from build123d import *

# Parameters (mm, degrees)
F1_DEPTH = 76.2
F2_W     = 17.6722221076
F2_H     = 9.8298916579
F2_W_2   = 18.5227831721
F3_DEPTH = 76.2
F4_R     = 3.4516477469
F4_R_2   = 3.5094678627
F5_DEPTH = 127
F6_R     = 3.428244009
F7_DEPTH = 127


with BuildPart() as f1:
    # F0 (on Right) → F1 (new body)
    with BuildSketch(Plane.YZ):
        with BuildLine():
            Line((-43.5515455902, 4.9651595764), (-39.2007894463, -3.8494697966))
            ThreePointArc((-39.2007894463, -3.8494697966), (59.7212641248, -33.7173735079), (95.7566574216, 63.1284564734))
            Line((95.7566574216, 63.1284564734), (82.136558344, 69.8877791238))
            Line((82.136558344, 69.8877791238), (86.031280458, 60.8586706221))
            ThreePointArc((86.031280458, 60.8586706221), (50.4707031722, -26.2634284737), (-35.969786346, 10.9233511612))
            Line((-35.969786346, 10.9233511612), (-43.5515455902, 4.9651595764))
        make_face()
    extrude(amount=F1_DEPTH)

    # F2 (on face) → F3 (join)
    with BuildSketch(Plane(origin=(0, -33.0492176978, -16.3125505187), x_dir=(1, 0, 0), z_dir=(0, -0.8967168388, -0.4426046894))):
        with Locations((8.8361110538, 18.8135146783)):
            Rectangle(F2_W, F2_H)
        with Locations((66.9386084139, 18.8135146783)):
            Rectangle(F2_W_2, F2_H)
    extrude(amount=F3_DEPTH)

    # F4 (on face) → F5 (cut)
    with BuildSketch(Plane.YZ.offset(76.2)):
        with Locations((-79.3107077479, -18.0164370686)):
            Circle(F4_R)
        with Locations((-95.9507897496, -26.2444168329)):
            Circle(F4_R_2)
    extrude(amount=-F5_DEPTH, mode=Mode.SUBTRACT)

    # F6 (on face) → F7 (cut)
    with BuildSketch(Plane.YZ.offset(76.2)):
        with Locations((-63.4221956134, -10.355903767)):
            Circle(F6_R)
    extrude(amount=-F7_DEPTH, mode=Mode.SUBTRACT)


solid = f1.part
Design review of the part built by this model. Coordinates are the model's own, in mm. A direction names the side the tool comes from. Coordinates: 2 decimals unless noted, no trailing zeros. Loops run counter-clockwise (first coordinate to the right, second up) from the corner with the lowest first, then second, coordinate; pieces in that order, holes last.
Item 1: Add section A-A (y = -97). Write out the cut boundary in (x, z).
Completed:
outline: (0, -32.38) - (17.67, -32.38) - (17.67, -29.59) - (0, -29.59) - close; (0, -22.9) - (17.67, -22.9) - (17.67, -21.42) - (0, -21.42) - close; (57.68, -32.38) - (76.2, -32.38) - (76.2, -29.59) - (57.68, -29.59) - close; (57.68, -22.9) - (76.2, -22.9) - (76.2, -21.42) - (57.68, -21.42) - close
Item 2: Clearance check with flat-ended pins moving along their axes: pin 1 (6 mm diameter, centred on y = -63.42, z = -10.36, fed in from -X); pin 2 (4 mm diameter, centred on x = 67, y = 39, fed in from +Z); pin 3 (6 mm diameter, centred on x = 10.5, z = 0, fed in from -Y); pin 4 (4 mm diameter, centred on x = 66.5, y = 54, fed in from +Z). State where each tip first meets the part, or that it passes through.
Completed:
pin 1: passes through
pin 2: stops at z = -29.33
pin 3: stops at y = -59.69
pin 4: stops at z = -23.7
Item 3: Add section B-B (y = -55). Write out the cut boundary in (x, z).
Completed:
outline: (0, -11.65) - (17.67, -11.65) - (17.67, -0.69) - (0, -0.69) - close; (57.68, -11.65) - (76.2, -11.65) - (76.2, -0.69) - (57.68, -0.69) - close
Item 4: Draft analysis for pull direction Z (two halves, no side actions). For faces 1 (the flat face through (66.809, -77.238, -11.662)), 2 (the flat face through (8.71, -72.89, -20.48)), 3 (the cylindrical face through (37.567, 51.822, -25.693)), state which applies: pulls with the +Z half, pulls with the -Z half, needs draft (parallel to the pull), parting line crosses it, or undercut.
Completed:
face 1: pulls with the +Z half
face 2: pulls with the -Z half
face 3: undercut
Item 5: Wall thickness on L1, parallel to Y at x = 12, z = -6.5; L2, parallel to Y at x = 17, z = -25; L3, parallel to Y at x = 67, z = -23: over which ranges is each line inside the solid? List them lowest first.
Completed:
L1: y = -66.78 to -44.57, -37.6 to -25.93, 76.92 to 89.93
L2: y = -104.26 to -99.23, -92.67 to -82.05, -21.04 to -2.36, 53.36 to 73.38
L3: y = -100.21 to -97.29, -94.61 to -78, -23.44 to -6.3, 57.3 to 75.77
Item 6: For faces 4 (the flat face through (37.567, -39.708, 7.986)), 5 (the flat face through (37.567, 84.057, 65.436)), list the 3-axis set-ups (+Z, -Z, +X, -X, +Y, -Y) from which the entire face can be reached by the end or side of a thin tool; tool diameter is ignored.
Completed:
face 4: +Z, +X, -X, -Y
face 5: +X, -X, -Y
